For this review, take the finished solid that the model builds, in its own axes (mm). A direction names the side the tool comes from. Coordinates: 2 decimals unless noted, no trailing zeros. Write each loop counter-clockwise with the first axis right and the second up, starting at its lowest first coordinate (ties: lowest second). Pieces come first, ordered by that corner, then holes.
```python
from build123d import *

# Parameters (mm, degrees)
SKETCH1_R           = 1
BOSS_EXTRUDE1_DEPTH = 9
BOSS_EXTRUDE2_DEPTH = 1
SKETCH3_R           = 0.916230728
CUT_EXTRUDE1_DEPTH  = 1
SKETCH5_OUTSIDE_W   = 8.162
SKETCH5_OUTSIDE_H   = 8.598
SKETCH5_OUTSIDE_R   = 1.19698552
CUT_EXTRUDE3_DEPTH  = 1
CUT_EXTRUDE3_DRAFT  = -30
FILLET1_R           = 0.2


with BuildPart() as part:
    # Sketch1 → Boss-Extrude1 (new body)
    with BuildSketch(Plane.XY):
        Circle(SKETCH1_R)
    extrude(amount=BOSS_EXTRUDE1_DEPTH)

    # Sketch2 → Boss-Extrude2 (add)
    with BuildSketch(Plane.XY.offset(9)):
        Polygon((0, 1.632320149), (-1.413630716, 0.816160075), (-1.413630716, -0.816160075), (0, -1.632320149), (1.413630716, -0.816160075), (1.413630716, 0.816160075), align=None)
    extrude(amount=BOSS_EXTRUDE2_DEPTH)

    # Sketch3 → Cut-Extrude1 (cut)
    with BuildSketch(Plane.XY.offset(10)):
        Circle(SKETCH3_R)
    extrude(amount=-CUT_EXTRUDE1_DEPTH, mode=Mode.SUBTRACT)


with BuildPart() as cut_extrude3_tool:
    # Sketch5 outside → Cut-Extrude3 (with draft: the straight prism first)
    with BuildSketch(Plane.XY.offset(10)):
        Rectangle(SKETCH5_OUTSIDE_W, SKETCH5_OUTSIDE_H)
        Circle(SKETCH5_OUTSIDE_R, mode=Mode.SUBTRACT)
    extrude(amount=-CUT_EXTRUDE3_DEPTH)
    # Cut-Extrude3: the draft: its side faces are tilted about the plane it starts from
    cut_extrude3_sides = [cut_extrude3_tool.faces().sort_by_distance(p)[0] for p in [
        (0, -4.299, 9.5),
        (4.081, 0, 9.5),
        (0, 4.299, 9.5),
        (-4.081, 0, 9.5),
        (-1.19698552, 0, 9.5),
    ]]
    draft(cut_extrude3_sides, Plane.XY.offset(10), CUT_EXTRUDE3_DRAFT)


with BuildPart() as part_1:
    add(part.part)

    # Cut-Extrude3: cut by cut_extrude3_tool
    add(cut_extrude3_tool.part, mode=Mode.SUBTRACT)

    # Fillet1
    fillet1_edges = [part_1.edges().sort_by_distance(p)[0] for p in [
        (-1, 0, 0),
    ]]
    fillet(fillet1_edges, radius=FILLET1_R)


solid = part_1.part
```
1) Consider section B-B (z = 4). Give the boundary of the cut face in (x, y), then the cut area to 3 significant figures.
2) The part is to be moulded in two halves that separate along X. For faces 4 (the face through (-0.717, -1.219, 9.239)), 5 (the face through (0, 0, 9)), 6 (the face through (0, 0, 0)), say which applies: pulls with the +X half, pulls with the -X half, needs draft (parallel to the pull), parting line crosses it, or undercut.
3) Consider section A-A (y = 0). Give the boundary of the cut face in (x, z).
4) Clearance check with flat-ended pins moving along their axes: P1, Ø1.6, axis at x = 0, y = 0, coming from the +Z side; P2, Ø1, axis at y = 0.5, z = 5.5, coming from the -X side. State where each tip first meets the part, or that it passes through.
5) For L1, parallel to Y at x = -0.05, z = 8.25; L2, parallel to Z at x = 0.75, y = 0.7; L3, parallel to Y at x = -0.6, z = 8, list the stretches that pass through material, from the lowest coordinate up.
6) Tool access review of faces 1 (the face through (0.7, -1.23, 9.24)), 2 (the face through (0, -1, 5)), 3 (the face through (-0.199, -0.894, 9.507)): name each direction out of +Z, -Z, +X, -X, +Y, -Y from which nothing blocks a thin tool from reaching the whole face with its end or side.
Results:
1. outline: circle Ø2 at (0, 0)
1. area: 3.14 mm2
2. face 4: pulls with the -X half
2. face 5: undercut
2. face 6: needs draft
3. outline: (-1.41, 9) - (-1, 9) - (-1, 0.2) arc R0.2 ccw to (-0.8, 0) - (0.8, 0) arc R0.2 ccw to (1, 0.2) - (1, 9) - (1.41, 9) - (1.41, 9.62) - (1.2, 10) - (0.92, 10) - (0.92, 9) - (-0.92, 9) - (-0.92, 10) - (-1.2, 10) - (-1.41, 9.62) - close
4. P1: stops at z = 9
4. P2: stops at x = -1
5. L1: y = -1 to 1
5. L2: z = 9 to 10
5. L3: y = -0.8 to 0.8
6. face 1: +Z, -Z, +X, -Y
6. face 2: -Z
6. face 3: +Z
